from build123d import *

# Parameters (mm, degrees)
SKETCH2_R           = 22.5
BOSS_EXTRUDE1_DEPTH = 5
SKETCH3_R           = 2
CUT_EXTRUDE1_DEPTH  = 5


with BuildPart() as part:
    # Sketch2 → Boss-Extrude1 (new body)
    with BuildSketch(Plane.XY):
        Circle(SKETCH2_R)
        Polygon((-22.5, 0), (-2.5, -22.360679775), (-24.860679775, -42.360679775), (-44.860679775, -20), align=None)
        Polygon((2.5, -22.360679775), (22.5, 0), (44.860679775, -20), (24.860679775, -42.360679775), align=None)
    extrude(amount=BOSS_EXTRUDE1_DEPTH)

    # Sketch3 → Cut-Extrude1 (cut)
    with BuildSketch(Plane(origin=(0, 0, 0), x_dir=(-1, 0, 0), z_dir=(0, 0, -1))):
        with Locations(Location((-37.800566479, -20.393446629, 0), (0, 0, 180))):
            Circle(SKETCH3_R)
        with Locations(Location((-22.893446629, -7.060113296, 0), (0, 0, 180))):
            Circle(SKETCH3_R)
        with Locations(Location((-9.560113296, -21.967233146, 0), (0, 0, 180))):
            Circle(SKETCH3_R)
        with Locations(Location((-24.467233146, -35.300566479, 0), (0, 0, 180))):
            Circle(SKETCH3_R)
        with Locations(Location((24.467233146, -35.300566479, 0), (0, 0, 180))):
            Circle(SKETCH3_R)
        with Locations(Location((37.800566479, -20.393446629, 0), (0, 0, 180))):
            Circle(SKETCH3_R)
        with Locations(Location((9.560113296, -21.967233146, 0), (0, 0, 180))):
            Circle(SKETCH3_R)
        with Locations(Location((22.893446629, -7.060113296, 0), (0, 0, 180))):
            Circle(SKETCH3_R)
    extrude(amount=-CUT_EXTRUDE1_DEPTH, mode=Mode.SUBTRACT)


solid = part.part
The listing builds one solid part. Answer for the finished solid, in the listing's coordinates (mm). A direction names the side the tool comes from. Coordinates: 2 decimals unless noted, no trailing zeros. Loops run counter-clockwise (first coordinate to the right, second up) from the corner with the lowest first, then second, coordinate; pieces in that order, holes last. Notation, with made-up numbers: (55.25, 40.25) -> (97.25, 40.25) arc R12 cw to (97.25, 60.25) -> close; hole circle Ø1 at (67.25, -35.75). An arc over 180 degrees is marked (long way). Write item = value, one per line. Start each with the question number.
1) A cutting plane is placed at B-B (y = -29). Give the vertices of the cut face in (x, z).
2) A tool of negligible diameter and unlimited length cuts with its end or side. For faces 4 (the face through (13.837, -32.501, 2.465)), 5 (the face through (-38.23, -18.44, 2.46)), from which of +Z, -Z, +X, -X, +Y, -Y can it reach the whole face along a straight path? Write none if from no direction.
3) The mould has two halves that part along X. Classify faces 1 (the face through (-21.971, -5.286, 2.465)), 2 (the face through (-34.72, -31.34, 2.46)), 3 (the face through (35.001, -31.024, 2.465)): released by +X, released by -X, zero draft, split by the parting line, or undercut.
4) Given pin 1 Ø1 at (y, z) = (-22.5, 1.5) entering from +X; pin 2 Ø1.5 at (x, z) = (4.5, 2.5) entering from -Y; pin 3 Ø3.5 at (x, y) = (-37.8, -20.39) entering from -Z; pin 4 Ø2 at (y, z) = (-12, 4) entering from -X, each flat-ended and moving along its own axis, determine where each tip first touches the part or whether it passes through.
5) A cutting plane is placed at C-C (x = 0). Give the vertices of the cut face in (y, z).
6) Straight lines are drawn through the part: line 1 (X direction, y = -34, z = 0.55); line 2 (X direction, y = -23, z = 0.9); line 3 (Y direction, x = -8, z = 1.1). For each, find the intervals that lie inside material, in ascending order. Write a range as from..to.
7) A cutting plane is placed at D-D (y = 4.5). Give the vertices of the cut face in (x, z).
8) A cutting plane is placed at A-A (z = 1.65). Count the separate pieces of the cut face and the enclosed holes in it, then the cut area to 3 significant figures.
Responses:
q1.outline = (-36.81, 0) -> (-9.92, 0) -> (-9.92, 5) -> (-36.81, 5) -> close; (9.92, 0) -> (36.81, 0) -> (36.81, 5) -> (9.92, 5) -> close
q2.face_4 = +Z, -Z, -Y
q2.face_5 = +Z, -Z
q3.face_1 = undercut
q3.face_2 = released by -X
q3.face_3 = released by +X
q4.pin_1 = 43.07
q4.pin_2 = -24.82
q4.pin_3 = through
q4.pin_4 = -37.03
q5.outline = (-22.5, 0) -> (22.5, 0) -> (22.5, 5) -> (-22.5, 5) -> close
q6.line_1 = -32.34..-25.99, -22.95..-15.51, 15.51..22.95, 25.99..32.34
q6.line_2 = -42.18..-11.27, -7.85..-3.21, 3.21..7.85, 11.27..42.18
q6.line_3 = -27.28..-23.22, -20.72..21.03
q7.outline = (-22.05, 0) -> (22.05, 0) -> (22.05, 5) -> (-22.05, 5) -> close
q8.separate_pieces = 1
q8.enclosed_holes = 8
q8.area = 3,050 mm²
